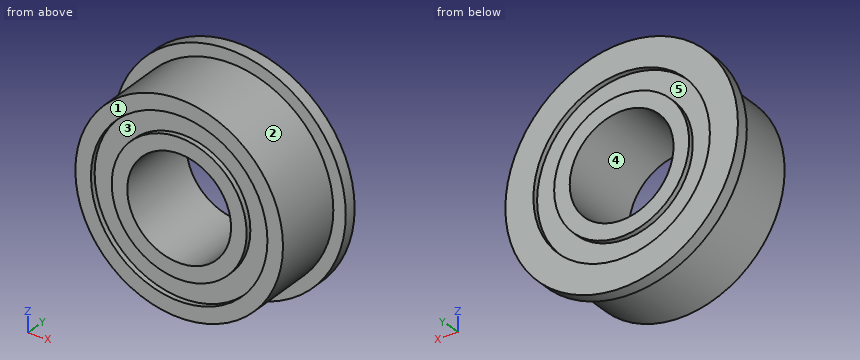
```python
from build123d import *

# Parameters (mm, degrees)
F2_R      = 5.6
F2_R_2    = 5
F3_DEPTH  = 0.6
F4_R      = 5
F4_R_2    = 4.25
F5_DEPTH  = 4
F6_R      = 3.25
F6_R_2    = 2.5
F7_DEPTH  = 4
F9_R      = 4.25
F9_R_2    = 3.25
F10_DEPTH = 1.75


with BuildPart() as f3:
    # F2 (on Front) → F3 (new body)
    with BuildSketch(Plane.XZ):
        Circle(F2_R)
        Circle(F2_R_2, mode=Mode.SUBTRACT)
    extrude(amount=F3_DEPTH)

    # F4 (on Front) → F5 (join)
    with BuildSketch(Plane.XZ):
        Circle(F4_R)
        Circle(F4_R_2, mode=Mode.SUBTRACT)
    extrude(amount=F5_DEPTH)



with BuildPart() as f7:
    # F6 (on Front) → F7 (new body)
    with BuildSketch(Plane.XZ):
        Circle(F6_R)
        Circle(F6_R_2, mode=Mode.SUBTRACT)
    extrude(amount=F7_DEPTH)


with BuildPart() as f3_1:
    add(f3.part)

    add(f7.part)  # F10 merges F7
    # F9 (on offset) → F10 (join, symmetric)
    with BuildSketch(Plane.XZ.offset(2)):
        Circle(F9_R)
        Circle(F9_R_2, mode=Mode.SUBTRACT)
    extrude(amount=F10_DEPTH, both=True)


solid = f3_1.part
```
Geometry check sheet. Reference: the model listing, model coordinates, mm. Face numbers are marked on the shaded views. A direction names the side the tool comes from. Coordinates: 2 decimals unless noted, no trailing zeros. Order: outer loops, then holes, each group sorted by start corner. A loop starts at its lowest first (then second) coordinate and runs counter-clockwise, first axis right, second up.
Item 1: Section check C-C (y = -3.5). Enter the section's corners in (x, z), plus the area to 3 significant figures.
Item 2: Section check B-B (x = 0). Enter the section's corners in (y, z), plus the area to 3 significant figures.
Item 3: Scan lines: line 1 along Z through (x, y) = (0, -3.9); line 2 along Z through (x, y) = (0, -3.5); line 3 along Z through (x, y) = (2, -2.1). Record each from-to range of solid material in increasing order.
Item 4: Section check A-A (z = 0). Enter the section's corners in (x, y), plus the area to 3 significant figures.
Item 5: Tool access check on the marked faces 4 and 5. Record the directions out of +Z, -Z, +X, -X, +Y, -Y that give a thin tool (end or side, any length) a straight path to the whole face; none if there is none.
Item 6: Section check D-D (z = 3). Enter the section's corners in (x, y), plus the area to 3 significant figures.
Item 7: Depth check by flat-ended pin: pin 1 (1.5 mm diameter, centred on x = 2, y = -3.5, fed in from +Z); pin 2 (2 mm diameter, centred on y = -2.5, z = 1.5, fed in from +X); pin 3 (1 mm diameter, centred on x = -2, y = -1, fed in from -Z). Enter the tip coordinate at first touch or a pass-through.
Item 8: Mould release check, pull along X, two halves, no side actions. Record for the marked faces 1, 2 and 3: released by +X, released by -X, zero draft, split by the parting line, or undercut.
Check sheet entries:
1. outline: circle Ø10 at (0, 0); hole circle Ø5 at (0, 0)
1. area: 58.9 mm2
2. outline: (-4, -5) - (-0.6, -5) - (-0.6, -5.6) - (0, -5.6) - (0, -4.25) - (-0.25, -4.25) - (-0.25, -3.25) - (0, -3.25) - (0, -2.5) - (-4, -2.5) - (-4, -3.25) - (-3.75, -3.25) - (-3.75, -4.25) - (-4, -4.25) - close; (-4, 2.5) - (0, 2.5) - (0, 3.25) - (-0.25, 3.25) - (-0.25, 4.25) - (0, 4.25) - (0, 5.6) - (-0.6, 5.6) - (-0.6, 5) - (-4, 5) - (-4, 4.25) - (-3.75, 4.25) - (-3.75, 3.25) - (-4, 3.25) - close
2. area: 19.7 mm2
3. line 1: z = -5 to -4.25, -3.25 to -2.5, 2.5 to 3.25, 4.25 to 5
3. line 2: z = -5 to -2.5, 2.5 to 5
3. line 3: z = -4.58 to -1.5, 1.5 to 4.58
4. outline: (-5.6, -0.6) - (-5, -0.6) - (-5, -4) - (-4.25, -4) - (-4.25, -3.75) - (-3.25, -3.75) - (-3.25, -4) - (-2.5, -4) - (-2.5, 0) - (-3.25, 0) - (-3.25, -0.25) - (-4.25, -0.25) - (-4.25, 0) - (-5.6, 0) - close; (2.5, -4) - (3.25, -4) - (3.25, -3.75) - (4.25, -3.75) - (4.25, -4) - (5, -4) - (5, -0.6) - (5.6, -0.6) - (5.6, 0) - (4.25, 0) - (4.25, -0.25) - (3.25, -0.25) - (3.25, 0) - (2.5, 0) - close
4. area: 19.7 mm2
5. face 4: +Y, -Y
5. face 5: +Y
6. outline: (-4.73, -0.6) - (-4, -0.6) - (-4, -4) - (-3.01, -4) - (-3.01, -3.75) - (-1.25, -3.75) - (-1.25, -4) - (1.25, -4) - (1.25, -3.75) - (3.01, -3.75) - (3.01, -4) - (4, -4) - (4, -0.6) - (4.73, -0.6) - (4.73, 0) - (3.01, 0) - (3.01, -0.25) - (1.25, -0.25) - (1.25, 0) - (-1.25, 0) - (-1.25, -0.25) - (-3.01, -0.25) - (-3.01, 0) - (-4.73, 0) - close
6. area: 31.1 mm2
7. pin 1: stops at z = 4.84
7. pin 2: stops at x = 4.97
7. pin 3: stops at z = -5.34
8. face 1: zero draft
8. face 2: split by the parting line
8. face 3: undercut
